Model file for the job. Use its own axes, mm. A direction names the side the tool comes from. Round coordinates to 2 decimals unless told otherwise and drop trailing zeros. Loops run counter-clockwise (first coordinate to the right, second up) from the corner with the lowest first, then second, coordinate; pieces in that order, holes last. Notation, with made-up numbers: M 74,73.25 L 93,73.25 A32 ccw 93,107.25 Z; hole C 65,77 d1. An arc over 180 degrees is marked long. Use a Markdown table: item, result. Add a question column.
Item 1: Saw through at C-C on x = -6.5. Write the cut outline in (y, z).
Item 2: Wall check: L1, parallel to Y at x = 0, z = -1.5; L2, parallel to Y at x = -0.5, z = 9.25; L3, parallel to Y at x = 7, z = 3.75. Give the ranges that are in metal, low to high. Write a range as from..to.
Item 3: Pin check, flat tips, straight feed: P1, Ø4, axis at x = 3, z = 14, coming from the +Y side; P2, Ø6, axis at x = 4.5, y = -20, coming from the +Z side; P3, Ø3, axis at y = -7.5, z = 0, coming from the -X side. Stop position of each tip, or through.
Item 4: Saw through at B-B on z = -4.5. Write the cut outline in (x, y).
Item 5: Two-plate mould, pull along Y, no slides. Class faces 5 (the flat face through (0, -20, -11)), 6 (the flat face through (0, -30, -2)), 7 (the cylindrical face through (0, -50, 11)): +Y half, -Y half, draft (parallel to the pull), parting line (faces both ways), or undercut.
Item 6: Tool access for faces 1 (the flat face through (-2, -5, 5.5)), 2 (the flat face through (-13, -30, 10)), 3 (the flat face through (13, -30, 10)), 4 (the flat face through (-9.5, -5, 0)): list every direction of +Z, -Z, +X, -X, +Y, -Y with a clear straight run to the whole face (end or side of a thin tool).
Item 7: Saw through at A-A on y = -5. Write the cut outline in (x, z), then the cut area to 3 significant figures.
Item 8: Saw through at D-D on y = -63. Write the cut outline in (x, z).
```python
from build123d import *

# Parameters (mm, degrees)
F0_W     = 19
F0_H     = 11
F1_DEPTH = 10
F2_W     = 34
F2_H     = 22
F3_DEPTH = 20
F5_DEPTH = 40
F7_DEPTH = 4
F8_R     = 1.5
F9_DEPTH = 16.501


with BuildPart() as f1:
    # F0 (on Front) → F1 (new body)
    with BuildSketch(Plane.XZ):
        Rectangle(F0_W, F0_H)
    extrude(amount=F1_DEPTH)

    # F2 (on face) → F3 (join)
    with BuildSketch(Plane.XZ.offset(10)):
        Rectangle(F2_W, F2_H)
    extrude(amount=F3_DEPTH)

    # F4 (on face) → F5 (join)
    with BuildSketch(Plane.XZ.offset(30)):
        with BuildLine():
            Line((17, 3.54129), (17, 8.737549))
            ThreePointArc((17, 8.737549), (0, 11), (-17, 8.737549))
            Line((-17, 8.737549), (-17, 3.54129))
            ThreePointArc((-17, 3.54129), (0, 6), (17, 3.54129))
        make_face()
    extrude(amount=F5_DEPTH)

    # F6 (on face) → F7 (join)
    with BuildSketch(Plane.XZ.offset(70)):
        with BuildLine():
            Line((-17, 8.737549), (-17, 3.54129))
            ThreePointArc((-17, 3.54129), (0, 6), (17, 3.54129))
            Line((17, 3.54129), (17, 8.737549))
            Line((17, 8.737549), (17, 14.934752))
            ThreePointArc((17, 14.934752), (0, 17), (-17, 14.934752))
            Line((-17, 14.934752), (-17, 8.737549))
        make_face()
    extrude(amount=F7_DEPTH)

    # F8 (on face) → F9 (cut, through all)
    with BuildSketch(Plane.XY.offset(5.5)):
        with Locations((0, -5)):
            Circle(F8_R)
    extrude(amount=-F9_DEPTH, mode=Mode.SUBTRACT)


solid = f1.part
```
Entries:
| question | item | result |
|---|---|---|
| 1 | outline | M -74,5.65 L -30,5.65 L -30,-11 L -10,-11 L -10,-5.5 L 0,-5.5 L 0,5.5 L -10,5.5 L -10,11 L -30,11 L -30,10.67 L -70,10.67 L -70,16.7 L -74,16.7 Z |
| 2 | L1 | -30..-6.5, -3.5..0 |
| 2 | L2 | -74..-10 |
| 2 | L3 | -30..0 |
| 3 | P1 | y = -70 |
| 3 | P2 | z = 11 |
| 3 | P3 | x = -9.5 |
| 4 | outline | M -17,-30 L 17,-30 L 17,-10 L 9.5,-10 L 9.5,0 L -9.5,0 L -9.5,-10 L -17,-10 Z; hole C 0,-5 d3 |
| 5 | face 5 | draft |
| 5 | face 6 | -Y half |
| 5 | face 7 | undercut |
| 6 | face 1 | +Z, +X, -X, +Y |
| 6 | face 2 | +Z, -X |
| 6 | face 3 | +Z, +X |
| 6 | face 4 | +Z, -Z, -X, +Y |
| 7 | outline | M -9.5,-5.5 L -1.5,-5.5 L -1.5,5.5 L -9.5,5.5 Z; M 1.5,-5.5 L 9.5,-5.5 L 9.5,5.5 L 1.5,5.5 Z |
| 7 | area | 176 mm2 |
| 8 | outline | M -17,3.54 A60 cw 17,3.54 L 17,8.74 A65 ccw -17,8.74 Z |
